The model under review builds one solid part; all positions refer to its coordinate system, in mm. A direction names the side the tool comes from. Round coordinates to 2 decimals unless told otherwise and drop trailing zeros. Order: outer loops, then holes, each group sorted by start corner. A loop starts at its lowest first (then second) coordinate and runs counter-clockwise, first axis right, second up. Notation, with made-up numbers: M 24,24 L 81,24 A23 cw 81,39 Z; hole C 6.25,-18.5 d9. An arc over 180 degrees is marked long. Answer as a JSON object with one key per item and string values. Group by question number.
1. Add section B-B on x = 0. State the section outline as (y, z) points.
2. To check wall thickness, follow probe 1 along X at (y, z) = (-7, 60); probe 2 along Y at (x, z) = (2, 106.5); probe 3 along Y at (x, z) = (0, 26.5). State the ranges of each line that lie inside material, in increasing order. Write a range as [from, to].
3. Machinability: for faces 1 (the face through (0, 19.05, 69)), 2 (the face through (-6.35, 18, 122)), 3 (the face through (0, 16.002, 69)), which of the approach directions +Z, -Z, +X, -X, +Y, -Y give a long, thin tool a straight path to every point of the face, cutting with its end or side? Answer none if there is none.
4. Add section C-C on y = 9.5. State the section outline as (x, z) points, and give its area (3 significant figures).
5. Add section D-D on z = 45. State the section outline as (x, y) points, and give its area (3 significant figures).
6. Add section A-A on x = -18.5. State the section outline as (y, z) points, and give its area (3 significant figures).
7. Mouldability with a two-part tool opening along Y and no side actions: class faces 4 (the face through (2, -17, 139.7)), 5 (the face through (-24.636, 18.326, 68.872)), 6 (the face through (0, -16.002, 69)) as released by +Y, released by -Y, zero draft, split by the parting line, or undercut.
```python
from build123d import *

# Parameters (mm, degrees)
BOSS_EXTRUDE1_DEPTH = 139.7
CUT_EXTRUDE1_DEPTH  = 3.048


with BuildPart() as part:
    # Sketch4 → Boss-Extrude1 (new body)
    with BuildSketch(Plane.XY):
        with BuildLine():
            Line((25.4, -16.51), (25.4, 16.51))
            ThreePointArc((25.4, 16.51), (24.656051224, 18.306051224), (22.86, 19.05))
            Line((22.86, 19.05), (-22.86, 19.05))
            ThreePointArc((-22.86, 19.05), (-24.656051224, 18.306051224), (-25.4, 16.51))
            Line((-25.4, 16.51), (-25.4, -16.51))
            ThreePointArc((-25.4, -16.51), (-24.656051224, -18.306051224), (-22.86, -19.05))
            Line((-22.86, -19.05), (22.86, -19.05))
            ThreePointArc((22.86, -19.05), (24.656051224, -18.306051224), (25.4, -16.51))
        make_face()
        with BuildLine():
            Line((22.352, 14.4018), (22.352, -14.4018))
            ThreePointArc((22.352, -14.4018), (21.883312271, -15.533312271), (20.7518, -16.002))
            Line((20.7518, -16.002), (-20.7518, -16.002))
            ThreePointArc((-20.7518, -16.002), (-21.883312271, -15.533312271), (-22.352, -14.4018))
            Line((-22.352, -14.4018), (-22.352, 14.4018))
            ThreePointArc((-22.352, 14.4018), (-21.883312271, 15.533312271), (-20.7518, 16.002))
            Line((-20.7518, 16.002), (20.7518, 16.002))
            ThreePointArc((20.7518, 16.002), (21.883312271, 15.533312271), (22.352, 14.4018))
        make_face(mode=Mode.SUBTRACT)
    extrude(amount=BOSS_EXTRUDE1_DEPTH)

    # Sketch7 → Cut-Extrude1 (cut)
    with BuildSketch(Plane(origin=(0, 19.05, 0), x_dir=(1, 0, 0), z_dir=(0, 1, 0))):
        with BuildLine():
            Line((-6.35, -20.240625), (-6.35, -14.684375))
            ThreePointArc((-6.35, -14.684375), (0, -8.334375), (6.35, -14.684375))
            Line((6.35, -14.684375), (6.35, -20.240625))
            ThreePointArc((6.35, -20.240625), (0, -26.590625), (-6.35, -20.240625))
        make_face()
        with BuildLine():
            Line((-6.35, -125.015625), (-6.35, -119.459375))
            ThreePointArc((-6.35, -119.459375), (0, -113.109375), (6.35, -119.459375))
            Line((6.35, -119.459375), (6.35, -125.015625))
            ThreePointArc((6.35, -125.015625), (0, -131.365625), (-6.35, -125.015625))
        make_face()
    extrude(amount=-CUT_EXTRUDE1_DEPTH, mode=Mode.SUBTRACT)


solid = part.part
```
Recorded:
{
 "1": {"outline": "M -19.05,0 L -16,0 L -16,139.7 L -19.05,139.7 Z; M 16,0 L 19.05,0 L 19.05,8.33 L 16,8.33 Z; M 16,26.59 L 19.05,26.59 L 19.05,113.11 L 16,113.11 Z; M 16,131.37 L 19.05,131.37 L 19.05,139.7 L 16,139.7 Z"},
 "2": {"probe 1": "x = [-25.4, -22.35], [22.35, 25.4]", "probe 2": "y = [-19.05, -16], [16, 19.05]", "probe 3": "y = [-19.05, -16]"},
 "3": {"face 1": "+Z, -Z, +X, -X, +Y", "face 2": "+Y", "face 3": "+Z, -Z"},
 "4": {"outline": "M -25.4,0 L -22.35,0 L -22.35,139.7 L -25.4,139.7 Z; M 22.35,0 L 25.4,0 L 25.4,139.7 L 22.35,139.7 Z", "area": "852 mm²"},
 "5": {"outline": "M -25.4,-16.51 A2.54 ccw -22.86,-19.05 L 22.86,-19.05 A2.54 ccw 25.4,-16.51 L 25.4,16.51 A2.54 ccw 22.86,19.05 L -22.86,19.05 A2.54 ccw -25.4,16.51 Z; hole M -22.35,-14.4 A1.6 ccw -20.75,-16 L 20.75,-16 A1.6 ccw 22.35,-14.4 L 22.35,14.4 A1.6 ccw 20.75,16 L -20.75,16 A1.6 ccw -22.35,14.4 Z", "area": "501 mm²"},
 "6": {"outline": "M -19.05,0 L -16,0 L -16,139.7 L -19.05,139.7 Z; M 16,0 L 19.05,0 L 19.05,139.7 L 16,139.7 Z", "area": "852 mm²"},
 "7": {"face 4": "zero draft", "face 5": "released by +Y", "face 6": "undercut"}
}
